Geometry: final body of the model. Coordinates: model frame, mm. A direction names the side the tool comes from. Coordinates: 2 decimals unless noted, no trailing zeros. Order: outer loops, then holes, each group sorted by start corner. A loop starts at its lowest first (then second) coordinate and runs counter-clockwise, first axis right, second up. Notation, with made-up numbers: (-31, 33.25) -> (-10, 33.25) arc R27 cw to (-10, 61.25) -> close; hole circle Ø8 at (-16, -22.75). An arc over 180 degrees is marked (long way). Use one line per item in the form item = value.
```python
from build123d import *

# Parameters (mm, degrees)
SKETCH1_W           = 13
SKETCH1_H           = 42
BOSS_EXTRUDE1_DEPTH = 7
SKETCH2_W           = 11
SKETCH2_H           = 3.6
CUT_EXTRUDE1_DEPTH  = 4
SKETCH3_R           = 1.7
CUT_EXTRUDE2_DEPTH  = 10


with BuildPart() as part:
    # Sketch1 → Boss-Extrude1 (new body)
    with BuildSketch(Plane.XY):
        with Locations((-19.139592704, 35.078039657)):
            Rectangle(SKETCH1_W, SKETCH1_H)
    extrude(amount=BOSS_EXTRUDE1_DEPTH)

    # Sketch2 → Cut-Extrude1 (cut)
    with BuildSketch(Plane(origin=(0, 0, 0), x_dir=(-1, 0, 0), z_dir=(0, 0, -1))):
        with Locations((19.139592704, 35.078039657)):
            Rectangle(SKETCH2_W, SKETCH2_H)
    extrude(amount=-CUT_EXTRUDE1_DEPTH, mode=Mode.SUBTRACT)

    # Sketch3 → Cut-Extrude2 (cut)
    with BuildSketch(Plane.XY):
        with Locations((-19.139592704, 42.078039657)):
            Circle(SKETCH3_R)
    extrude(amount=CUT_EXTRUDE2_DEPTH, mode=Mode.SUBTRACT)


solid = part.part
```
1) Section A-A, the plane y = 35. Output: boundary loops of the cut face in (x, z).
Results found:
outline = (-25.64, 0) -> (-24.64, 0) -> (-24.64, 4) -> (-13.64, 4) -> (-13.64, 0) -> (-12.64, 0) -> (-12.64, 7) -> (-25.64, 7) -> close
2) Section B-B, the plane z = 2.25. Output: boundary loops of the cut face in (x, y), and give its area (3 significant figures).
Results found:
outline = (-25.64, 14.08) -> (-12.64, 14.08) -> (-12.64, 56.08) -> (-25.64, 56.08) -> close; hole (-24.64, 33.28) -> (-13.64, 33.28) -> (-13.64, 36.88) -> (-24.64, 36.88) -> close; hole circle Ø3.4 at (-19.14, 42.08)
area = 497 mm2
3) Section C-C, the plane x = -18.25. Output: boundary loops of the cut face in (y, z), and give its area (3 significant figures).
Results found:
outline = (14.08, 0) -> (33.28, 0) -> (33.28, 4) -> (36.88, 4) -> (36.88, 0) -> (40.63, 0) -> (40.63, 7) -> (14.08, 7) -> close; (43.53, 0) -> (56.08, 0) -> (56.08, 7) -> (43.53, 7) -> close
area = 259 mm2
4) Material intervals for probe 1 along Y at (x, z) = (-17.75, 2); probe 2 along Y at (x, z) = (-14.25, 1.75); probe 3 along X at (y, z) = (42, 3.75), sorted ascending. Write a range as from..to.
Results found:
probe_1 = 14.08..33.28, 36.88..41.1, 43.06..56.08
probe_2 = 14.08..33.28, 36.88..56.08
probe_3 = -25.64..-20.84, -17.44..-12.64
5) Access query for faces 4 (the flat face through (-19, 35, 7)), 5 (the flat face through (-13.64, 35, 2)). Directions: +Z, -Z, +X, -X, +Y, -Y. A direction counts if a zero-diameter tool reaches every point of the face in a straight line with its end or side. Return the directions, or none.
Results found:
face_4 = +Z, +X, -X, +Y, -Y
face_5 = -Z
6) Pull-direction query (X, two-part tool) for faces 1 (the flat face through (-19, 40, 0)), 2 (the flat face through (-19, 33.278, 2)), 3 (the flat face through (-25.64, 35, 3)); classes: released by +X, released by -X, zero draft, split by the parting line, or undercut.
Results found:
face_1 = zero draft
face_2 = undercut
face_3 = released by -X
7) Section D-D, the plane y = 41. Output: boundary loops of the cut face in (x, z), and give its area (3 significant figures).
Results found:
outline = (-25.64, 0) -> (-20.45, 0) -> (-20.45, 7) -> (-25.64, 7) -> close; (-17.83, 0) -> (-12.64, 0) -> (-12.64, 7) -> (-17.83, 7) -> close
area = 72.6 mm2
8) Contact query for a flat-ended pin moving along its axis: P1, Ø1.1, axis at x = -21, y = 34.5, coming from the -Z side. Output: stop coordinate, or through.
Results found:
P1 = 4
